Verification items for the finished model (mm, model axes). A direction names the side the tool comes from. Give positions to 0.01 mm unless a question says otherwise; leave off trailing zeros. Write each loop counter-clockwise with the first axis right and the second up, starting at its lowest first coordinate (ties: lowest second). Pieces come first, ordered by that corner, then holes. Notation, with made-up numbers: (67, 11.25) -> (120, 11.25) arc R24 ccw to (120, 30.25) -> close; hole circle Ø10 at (83, 10). An arc over 180 degrees is marked (long way). Answer as CSV lines item,"result". Start each with the question number.
1) Mould release check, pull along Z, two halves, no side actions. Record for faces 3 (the flat face through (5.2, -22, -1.9)), 4 (the cylindrical face through (-5.8, -8.41, 13.11)), 5 (the flat face through (4.525, -19.535, -2.662)): released by +Z, released by -Z, zero draft, split by the parting line, or undercut.
2) Material ranges on L1, parallel to Z at x = 0, y = -13; L2, parallel to X at y = -3, z = 9; L3, parallel to Y at x = 6.75, z = -5, recorded low to high.
3) Sectioned sample at A-A on x = 0. Record the cut outline in (y, z), and give its area (3 significant figures).
4) Sectioned sample at C-C on y = -6.5. Record the cut outline in (x, z).
5) Sectioned sample at B-B on y = -18.5. Record the cut outline in (x, z).
6) Tool access check on faces 1 (the flat face through (0, -20, -5.25)), 2 (the cylindrical face through (2.5, -8.381, -1.917)). Record the directions out of +Z, -Z, +X, -X, +Y, -Y that give a thin tool (end or side, any length) a straight path to the whole face; none if there is none.
7) Gauge pin test, flat ends, axial feed: pin 1 Ø2.5 at (x, y) = (-1.5, -19.5) entering from -Z; pin 2 Ø4 at (y, z) = (-6, 5.5) entering from +X; pin 3 Ø5.5 at (x, y) = (0.5, -18.5) entering from +Z. Record the tip position at first contact, or that the pin passes through.
```python
from build123d import *

# Parameters (mm, degrees)
F2_R        = 5
F3_DEPTH    = 15
F4_T1_DEPTH = 31.851779741
F6_DEPTH    = 5
F7_D        = 6.3
F8_R        = 2


# Not quite as in the source:
# - a fillet or chamfer that OpenCascade refuses, or shapes differently, is made with other operations: its cross-section is extruded or revolved along the edge and cut away or added


with BuildPart() as f1:
    # F0 (on Right) → F1 (revolve)
    with BuildSketch(Plane.YZ):
        Polygon((-22, 0), (0, 0), (0, 15), (-15, 15), (-15, 8), (-22, 8), align=None)
    revolve(axis=Axis((0, -11, 0), (0, -1, 0)))

    # F2 (on face) → F3 (cut)
    with BuildSketch(Plane(origin=(0, 0, 0), x_dir=(-1, 0, 0), z_dir=(0, 1, 0))):
        with Locations((0, 15)):
            Circle(F2_R)
        with Locations((-14.2658477444, 4.6352549156)):
            Circle(F2_R)
        with Locations((-8.8167787844, -12.1352549156)):
            Circle(F2_R)
        with Locations((8.8167787844, -12.1352549156)):
            Circle(F2_R)
        with Locations((14.2658477444, 4.6352549156)):
            Circle(F2_R)
    extrude(amount=-F3_DEPTH, mode=Mode.SUBTRACT)

    # F4: fillet of radius 3 on 10 edges, made by hand

    # F4_s2 → F4_t1 (cut)
    with BuildSketch(Plane.XZ.offset(-8.4258898705)):
        with BuildLine():
            ThreePointArc((14.5487698044, -3.6514787659), (14.2786844682, -1.4956481826), (12.6240778064, -0.0875187896))
            ThreePointArc((12.6240778064, -0.0875187896), (13.7969148622, -0.3427067106), (14.9967749751, -0.3110311036))
            ThreePointArc((14.9967749751, -0.3110311036), (14.8668911251, -1.993877698), (14.5487698044, -3.6514787659))
        make_face()
        with BuildLine():
            ThreePointArc((10.1616512299, 7.4910509465), (10.6725784478, 9.6028049498), (9.6239166514, 11.5056607062))
            ThreePointArc((9.6239166514, 11.5056607062), (10.855595668, 10.3516202931), (11.94982632, 9.0665126108))
            ThreePointArc((11.94982632, 9.0665126108), (10.9605006431, 8.3868786361), (10.1616512299, 7.4910509465))
        make_face()
        with BuildLine():
            ThreePointArc((1.0230544424, -14.9650713198), (2.9899102079, -14.0420166136), (3.8178192654, -12.0332562533))
            ThreePointArc((3.8178192654, -12.0332562533), (3.9375477121, -13.2275479821), (4.3384501703, -14.3588944602))
            ThreePointArc((4.3384501703, -14.3588944602), (2.6978316338, -14.755395775), (1.0230544424, -14.9650713198))
        make_face()
        with BuildLine():
            ThreePointArc((10.2645357375, -7.3494425703), (12.4308183364, -7.1827953553), (13.9164873867, -5.5974439539))
            ThreePointArc((13.9164873867, -5.5974439539), (13.1995394795, -7.1254584084), (12.3154653113, -8.5632537137))
            ThreePointArc((12.3154653113, -8.5632537137), (11.3633765438, -7.8323675302), (10.2645357375, -7.3494425703))
        make_face()
        with BuildLine():
            ThreePointArc((-13.9164873867, -5.5974439539), (-12.4308183364, -7.1827953553), (-10.2645357375, -7.3494425703))
            ThreePointArc((-10.2645357375, -7.3494425703), (-11.3633765438, -7.8323675302), (-12.3154653113, -8.5632537137))
            ThreePointArc((-12.3154653113, -8.5632537137), (-13.1995394795, -7.1254584084), (-13.9164873867, -5.5974439539))
        make_face()
        with BuildLine():
            ThreePointArc((-3.8178192654, -12.0332562533), (-2.9899102079, -14.0420166136), (-1.0230544424, -14.9650713198))
            ThreePointArc((-1.0230544424, -14.9650713198), (-2.6978316338, -14.755395775), (-4.3384501703, -14.3588944602))
            ThreePointArc((-4.3384501703, -14.3588944602), (-3.9375477121, -13.2275479821), (-3.8178192654, -12.0332562533))
        make_face()
        with BuildLine():
            ThreePointArc((-12.6240778064, -0.0875187896), (-14.2786844682, -1.4956481826), (-14.5487698044, -3.6514787659))
            ThreePointArc((-14.5487698044, -3.6514787659), (-14.8668911251, -1.993877698), (-14.9967749751, -0.3110311036))
            ThreePointArc((-14.9967749751, -0.3110311036), (-13.7969148622, -0.3427067106), (-12.6240778064, -0.0875187896))
        make_face()
        with BuildLine():
            ThreePointArc((-10.1616512299, 7.4910509465), (-10.6725784478, 9.6028049498), (-9.6239166514, 11.5056607062))
            ThreePointArc((-9.6239166514, 11.5056607062), (-10.855595668, 10.3516202931), (-11.94982632, 9.0665126108))
            ThreePointArc((-11.94982632, 9.0665126108), (-10.9605006431, 8.3868786361), (-10.1616512299, 7.4910509465))
        make_face()
        with BuildLine():
            ThreePointArc((7.9685797912, 12.7083333333), (5.8348021081, 13.1176552016), (3.9842898956, 11.9791666667))
            ThreePointArc((3.9842898956, 11.9791666667), (4.5894146126, 13.0157435868), (4.9300664859, 14.1666666667))
            ThreePointArc((4.9300664859, 14.1666666667), (6.4904123885, 13.5231115882), (7.9685797912, 12.7083333333))
        make_face()
        with BuildLine():
            ThreePointArc((-3.9842898956, 11.9791666667), (-5.8348021081, 13.1176552016), (-7.9685797912, 12.7083333333))
            ThreePointArc((-7.9685797912, 12.7083333333), (-6.4904123885, 13.5231115882), (-4.9300664859, 14.1666666667))
            ThreePointArc((-4.9300664859, 14.1666666667), (-4.5894146126, 13.0157435868), (-3.9842898956, 11.9791666667))
        make_face()
    extrude(amount=F4_T1_DEPTH, mode=Mode.SUBTRACT)

    # F5 (on face) → F6 (cut)
    with BuildSketch(Plane.XZ.offset(22)):
        Polygon((3.0310889132, 5.25), (-3.0310889132, 5.25), (-6.0621778265, 0), (-3.0310889132, -5.25), (3.0310889132, -5.25), (6.0621778265, 0), align=None)
    extrude(amount=-F6_DEPTH, mode=Mode.SUBTRACT)

    # F7 (through all)
    with Locations(Plane.XZ.offset(22)):
        with Locations((0, 0)):
            Hole(F7_D / 2)

    # F8
    f8_edges = [f1.edges().sort_by_distance(p)[0] for p in [
        (-8.816779, 0, 12.135255),
        (-5.834802, 0, 13.117655),
        (-10.672578, 0, 9.602805),
        (0, 0, 10),
        (-9.510565, 0, 3.09017),
        (5.834802, 0, 13.117655),
        (-14.278684, 0, -1.495648),
        (8.816779, 0, 12.135255),
        (-14.265848, 0, -4.635255),
        (10.672578, 0, 9.602805),
        (-12.430818, 0, -7.182795),
        (9.510565, 0, 3.09017),
        (-5.877853, 0, -8.09017),
        (14.278684, 0, -1.495648),
        (-2.98991, 0, -14.042017),
        (14.265848, 0, -4.635255),
        (0, 0, -15),
        (12.430818, 0, -7.182795),
        (2.98991, 0, -14.042017),
        (5.877853, 0, -8.09017),
    ]]
    fillet(f8_edges, radius=F8_R)


solid = f1.part
```
Ans:
1,face 3,"zero draft"
1,face 4,"released by +Z"
1,face 5,"undercut"
2,L1,"z = -15 to -3.15, 3.15 to 10"
2,L2,"x = -10.69 to 10.69"
2,L3,"y = -15 to 0"
3,outline,"(-22, -8) -> (-15, -8) -> (-15, -15) -> (-2, -15) arc R2 ccw to (0, -13) -> (0, -3.15) -> (-17, -3.15) -> (-17, -5.25) -> (-22, -5.25) -> close; (-22, 5.25) -> (-17, 5.25) -> (-17, 3.15) -> (0, 3.15) -> (0, 8) arc R2 ccw to (-2, 10) -> (-15, 10) -> (-15, 8) -> (-22, 8) -> close"
3,area,"326 mm²"
4,outline,"(-14.55, -3.65) arc R15 ccw to (-13.92, -5.6) arc R3 ccw to (-10.26, -7.35) arc R5 cw to (-3.82, -12.03) arc R3 ccw to (-1.02, -14.97) arc R15 ccw to (1.02, -14.97) arc R3 ccw to (3.82, -12.03) arc R5 cw to (10.26, -7.35) arc R3 ccw to (13.92, -5.6) arc R15 ccw to (14.55, -3.65) arc R3 ccw to (12.62, -0.09) arc R5 cw to (10.16, 7.49) arc R3 ccw to (9.62, 11.51) arc R15 ccw to (7.97, 12.71) arc R3 ccw to (3.98, 11.98) arc R5 cw to (-3.98, 11.98) arc R3 ccw to (-7.97, 12.71) arc R15 ccw to (-9.62, 11.51) arc R3 ccw to (-10.16, 7.49) arc R5 cw to (-12.62, -0.09) arc R3 ccw to start; hole circle Ø6.3 at (0, 0)"
5,outline,"circle Ø16 at (0, 0); hole (-6.06, 0) -> (-3.03, -5.25) -> (3.03, -5.25) -> (6.06, 0) -> (3.03, 5.25) -> (-3.03, 5.25) -> close"
6,face 1,"-Y"
6,face 2,"+Y, -Y"
7,pin 1,"stops at z = -8"
7,pin 2,"stops at x = 10.17"
7,pin 3,"stops at z = 8"
